Source: CAD feature listing. Evaluate the final solid. Frame: model axes, mm. A direction names the side the tool comes from. Round coordinates to 2 decimals unless told otherwise and drop trailing zeros. Write each loop counter-clockwise with the first axis right and the second up, starting at its lowest first coordinate (ties: lowest second). Pieces come first, ordered by that corner, then holes. Notation, with made-up numbers: M -29,36.25 L -21,36.25 A24 cw -21,46.25 Z; hole C 74.5,75.5 d4. An arc over 180 degrees is marked long. Answer in a Markdown table with one row per item.
from build123d import *

# Parameters (mm, degrees)
F0_W     = 50.8
F0_H     = 88.9
F1_DEPTH = 31.75
F2_W     = 25.4
F2_H     = 82.55
F3_DEPTH = 44.45
F4_W     = 25.4
F4_H     = 25.4
F5_DEPTH = 25.4


with BuildPart() as f1:
    # F0 (on Front) → F1 (new body)
    with BuildSketch(Plane.XZ):
        Rectangle(F0_W, F0_H)
    extrude(amount=F1_DEPTH)

    # F2 (on face) → F3 (cut)
    with BuildSketch(Plane.YZ.offset(25.4)):
        with Locations((-19.05, 3.175)):
            Rectangle(F2_W, F2_H)
    extrude(amount=-F3_DEPTH, mode=Mode.SUBTRACT)

    # F4 (on face) → F5 (cut)
    with BuildSketch(Plane(origin=(-25.4, 0, 0), x_dir=(0, -1, 0), z_dir=(-1, 0, 0))):
        with Locations((19.05, 31.75)):
            Rectangle(F4_W, F4_H)
    extrude(amount=-F5_DEPTH, mode=Mode.SUBTRACT)


solid = f1.part
Q1. Material intervals for probe 1 along Y at (x, z) = (23, -0.5); probe 2 along Z at (x, y) = (-6, -24); probe 3 along Z at (x, y) = (-20, -19.5), sorted ascending.
Solutions:
| item | result |
|---|---|
| probe 1 | y = -6.35 to 0 |
| probe 2 | z = -44.45 to -38.1 |
| probe 3 | z = -44.45 to 19.05 |
Q2. Contact query for flat-ended pins moving along their axis: pin 1 Ø8 at (x, z) = (1, -20) entering from -Y; pin 2 Ø7 at (x, y) = (-22, -14) entering from +Z; pin 3 Ø5 at (y, z) = (-14, 2.5) entering from +X; pin 4 Ø6 at (x, z) = (-9, -12) entering from +Y. Output: stop coordinate, or through.
Solutions:
| item | result |
|---|---|
| pin 1 | stops at y = -6.35 |
| pin 2 | stops at z = 19.05 |
| pin 3 | stops at x = -19.05 |
| pin 4 | stops at y = 0 |
Q3. Access query for faces 1 (the flat face through (-19.05, -19, -9)), 2 (the flat face through (-21, -31.75, -27)), 3 (the flat face through (-22, -19, 19.05)). Directions: +Z, -Z, +X, -X, +Y, -Y. A direction counts if a zero-diameter tool reaches every point of the face in a straight line with its end or side. Return the directions, or none.
Solutions:
| item | result |
|---|---|
| face 1 | +Z, +X, -Y |
| face 2 | +Z, -Z, +X, -X, -Y |
| face 3 | +Z, +X, -X, -Y |
Q4. Section B-B (y = -14.5). Return loops of the section in (x, z).
Solutions:
| item | result |
|---|---|
| outline | M -25.4,-44.45 L 25.4,-44.45 L 25.4,-38.1 L -19.05,-38.1 L -19.05,19.05 L -25.4,19.05 Z |
Q5. Section A-A (x = 1). Return loops of the section in (y, z).
Solutions:
| item | result |
|---|---|
| outline | M -31.75,-44.45 L 0,-44.45 L 0,44.45 L -6.35,44.45 L -6.35,-38.1 L -31.75,-38.1 Z |
Q6. Section C-C (z = 37.5). Return loops of the section in (x, y).
Solutions:
| item | result |
|---|---|
| outline | M -25.4,-6.35 L 25.4,-6.35 L 25.4,0 L -25.4,0 Z |
